```python
from build123d import *

# Parameters (mm, degrees)
SKETCH1_R           = 39.37
BOSS_EXTRUDE1_DEPTH = 13.335
SKETCH2_R           = 4.7625
CUT_EXTRUDE1_DEPTH  = 88.401931472
BOSS_EXTRUDE2_START = -2.54
SKETCH4_R           = 39.37
BOSS_EXTRUDE2_DEPTH = 2.54
SKETCH5_R           = 3.4925
CUT_EXTRUDE2_DEPTH  = 2.54
SKETCH6_R           = 15.24
CUT_EXTRUDE3_DEPTH  = 2.54


with BuildPart() as part:
    # Sketch1 → Boss-Extrude1 (new body)
    with BuildSketch(Plane(origin=(0, 0, 0), x_dir=(1, 0, 0), z_dir=(0, 1, 0))):
        with BuildLine():
            Line((-19.05, 57.15), (19.05, 57.15))
            Line((19.05, 57.15), (19.05, 41.562193157))
            ThreePointArc((19.05, 41.562193157), (45.72, 0), (19.05, -41.562193157))
            Line((19.05, -41.562193157), (19.05, -57.15))
            Line((19.05, -57.15), (-19.05, -57.15))
            Line((-19.05, -57.15), (-19.05, -41.562193157))
            ThreePointArc((-19.05, -41.562193157), (-45.72, 0), (-19.05, 41.562193157))
            Line((-19.05, 41.562193157), (-19.05, 57.15))
        make_face()
        with Locations(Location((0, 0, 0), (0, 0, 270))):
            Circle(SKETCH1_R, mode=Mode.SUBTRACT)
    extrude(amount=BOSS_EXTRUDE1_DEPTH)

    # Sketch2 → Cut-Extrude1 (cut, through all)
    with BuildSketch(Plane.ZY.offset(19.05)):
        with BuildLine():
            ThreePointArc((45.4025, 6.6675), (50.165, 1.905), (54.9275, 6.6675))
            Line((54.9275, 6.6675), (45.4025, 6.6675))
        make_face()
        with BuildLine():
            Line((45.4025, 6.6675), (54.9275, 6.6675))
            ThreePointArc((54.9275, 6.6675), (50.165, 11.43), (45.4025, 6.6675))
        make_face()
        with Locations((-50.165, 6.6675)):
            Circle(SKETCH2_R)
    extrude(amount=-CUT_EXTRUDE1_DEPTH, mode=Mode.SUBTRACT)

    # Sketch4 → Boss-Extrude2 (add)
    with BuildSketch(Plane(origin=(0, 13.335, 0), x_dir=(1, 0, 0), z_dir=(0, 1, 0)).offset(BOSS_EXTRUDE2_START)):
        with Locations(Location((0, 0, 0), (0, 0, 270))):
            Circle(SKETCH4_R)
    extrude(amount=BOSS_EXTRUDE2_DEPTH)

    # Sketch5 → Cut-Extrude2 (cut)
    with BuildSketch(Plane(origin=(0, 13.335, 0), x_dir=(1, 0, 0), z_dir=(0, 1, 0))):
        with Locations(Location((30.48, 0, 0), (0, 0, 270))):
            Circle(SKETCH5_R)
        with Locations(Location((-30.48, 0, 0), (0, 0, 270))):
            Circle(SKETCH5_R)
    extrude(amount=-CUT_EXTRUDE2_DEPTH, mode=Mode.SUBTRACT)

    # Sketch6 → Cut-Extrude3 (cut)
    with BuildSketch(Plane(origin=(0, 13.335, 0), x_dir=(1, 0, 0), z_dir=(0, 1, 0))):
        with Locations(Location((0, 0, 0), (0, 0, 270))):
            Circle(SKETCH6_R)
    extrude(amount=-CUT_EXTRUDE3_DEPTH, mode=Mode.SUBTRACT)


solid = part.part
```
Check sheet for the modelled part. Datum: model origin and axes. Units: mm. A direction names the side the tool comes from. Round coordinates to 2 decimals unless told otherwise and drop trailing zeros. Order: outer loops, then holes, each group sorted by start corner. A loop starts at its lowest first (then second) coordinate and runs counter-clockwise, first axis right, second up.
1) Mould release check, pull along X, two halves, no side actions. Record for faces 1 (the cylindrical face through (-33.89, 12.08, -0.76)), 2 (the cylindrical face through (-45.714, 6.574, 0.73)), 3 (the flat face through (0, 7, 57.15)): +X half, -X half, draft (parallel to the pull), parting line (faces both ways), or undercut.
2) Section check D-D (x = 30.48). Record the boundary of the cut face in (y, z) (1 decimal).
3) Scan lines: line 1 (X direction, y = 12.65, z = 0); line 2 (X direction, y = 11.75, z = -46); line 3 (Y direction, x = 20, z = -28) (3 decimals). Record each from-to range of solid material in increasing order.
4) Section check B-B (x = -14). Give the number of separate pieces and of enclosed holes in the cut face, and give its area (3 significant figures).
5) Section check C-C (z = 13). Record the boundary of the cut face in (x, y) (3 decimals), and give its area (3 significant figures).
6) Section check A-A (y = 9.25). Record the boundary of the cut face in (x, z), and give its area (3 significant figures).
7) Go/stop test with flat-tipped pins: pin 1 Ø12 at (x, z) = (-0.5, -24.5) entering from -Y (3 decimals); pin 2 Ø5.5 at (y, z) = (6.67, -50.16) entering from -X; pin 3 Ø6 at (y, z) = (4.5, -42.5) entering from +X; pin 4 Ø1.5 at (y, z) = (8, 41.5) entering from -X. Record where each tip stops, or that it passes through.
8) Tool access check on faces 4 (the cylindrical face through (-38.434, 5.322, -8.535)), 5 (the flat face through (19.05, 4, -46)), 6 (the flat face through (-19.05, 4, 46)), 7 (the flat face through (19.05, 10, 46)). Record the directions out of +Z, -Z, +X, -X, +Y, -Y that give a thin tool (end or side, any length) a straight path to the whole face; none if there is none.
Result:
1. face 1: undercut
1. face 2: -X half
1. face 3: draft
2. outline: (0, -34.1) - (13.3, -34.1) - (13.3, -3.5) - (10.8, -3.5) - (10.8, -24.9) - (0, -24.9) - close; (0, 24.9) - (10.8, 24.9) - (10.8, 3.5) - (13.3, 3.5) - (13.3, 34.1) - (0, 34.1) - close
3. line 1: x = -45.72 to -33.97, -26.99 to -15.24, 15.24 to 26.99, 33.97 to 45.72
3. line 2: x = -19.05 to 19.05
3. line 3: y = 10.795 to 13.335
4. separate pieces: 2
4. enclosed holes: 2
4. area: 557 mm2
5. outline: (-43.833, 0) - (-37.162, 0) - (-37.162, 10.795) - (-7.953, 10.795) - (-7.953, 13.335) - (-43.833, 13.335) - close; (7.953, 10.795) - (37.162, 10.795) - (37.162, 0) - (43.833, 0) - (43.833, 13.335) - (7.953, 13.335) - close
5. area: 326 mm2
6. outline: (-19.05, -57.15) - (19.05, -57.15) - (19.05, -54.17) - (-19.05, -54.17) - close; (-19.05, -46.16) - (19.05, -46.16) - (19.05, -41.56) arc R45.72 ccw to (19.05, 41.56) - (19.05, 46.16) - (-19.05, 46.16) - (-19.05, 41.56) arc R45.72 ccw to (-19.05, -41.56) - close; (-19.05, 54.17) - (19.05, 54.17) - (19.05, 57.15) - (-19.05, 57.15) - close; hole circle Ø78.74 at (0, 0)
6. area: 2,060 mm2
7. pin 1: stops at y = 10.795
7. pin 2: passes through
7. pin 3: stops at x = 23.02
7. pin 4: stops at x = -20.73
8. face 4: -Y
8. face 5: -Z, +X, +Y, -Y
8. face 6: +Z, -X, +Y, -Y
8. face 7: +Z, +X, +Y, -Y
